```python
from build123d import *

# Parameters (mm, degrees)
F0_R     = 12.7
F1_DEPTH = 19.05
F2_DEPTH = 6.35
F0_R_2   = 4.7625
F3_DEPTH = 9.525


with BuildPart() as f1:
    # F0 (on Front) → F1 (new body)
    with BuildSketch(Plane.XZ):
        with BuildLine():
            Line((21.9405616204, -3.5443449016), (22.1211236947, -2.1462785193))
            ThreePointArc((22.1211236947, -2.1462785193), (22.199015734, -1.0743953845), (22.225, 0))
            Line((22.225, 0), (21.5661626468, 5.3713363041))
            ThreePointArc((21.5661626468, 5.3713363041), (-1.3190436674, 22.1858231491), (-22.0506835685, 2.7781251166))
            ThreePointArc((-22.0506835685, 2.7781251166), (-22.225, 1.708e-07), (-22.0506836112, -2.7781247776))
            ThreePointArc((-22.0506836112, -2.7781247776), (-0.3870465512, -22.2216295525), (21.9405616204, -3.5443449016))
        make_face()
        Circle(F0_R, mode=Mode.SUBTRACT)
    extrude(amount=F1_DEPTH)

    # F0 (on Front) → F2 (join)
    with BuildSketch(Plane.XZ):
        with BuildLine():
            ThreePointArc((-22.0506835685, 2.7781251166), (-1.3190436674, 22.1858231491), (21.5661626468, 5.3713363041))
            Line((21.5661626468, 5.3713363041), (15.7569112616, 52.732711177))
            ThreePointArc((15.7569112616, 52.732711177), (15.8454503135, 51.7681577149), (15.875, 50.8))
            ThreePointArc((15.875, 50.8), (-0.9941387366, 34.9561585096), (-15.7504882737, 52.784375))
            Line((-15.7504882737, 52.784375), (-22.0506835685, 2.7781251166))
        make_face()
        with BuildLine():
            Line((15.8726570063, -50.5272646713), (21.9405616204, -3.5443449016))
            ThreePointArc((21.9405616204, -3.5443449016), (-0.3870465512, -22.2216295525), (-22.0506836112, -2.7781247776))
            Line((-22.0506836112, -2.7781247776), (-15.7504882737, -52.784375))
            ThreePointArc((-15.7504882737, -52.784375), (-1.1302070867, -34.9652831746), (15.8726570063, -50.5272646713))
        make_face()
    extrude(amount=F2_DEPTH)

    # F0 (on Front) → F3 (join)
    with BuildSketch(Plane.XZ):
        with BuildLine():
            ThreePointArc((15.875, 50.8), (15.8454503135, 51.7681577149), (15.7569112616, 52.732711177))
            ThreePointArc((15.7569112616, 52.732711177), (0.0260307769, 66.6749786582), (-15.7504882737, 52.784375))
            ThreePointArc((-15.7504882737, 52.784375), (-0.9941387366, 34.9561585096), (15.875, 50.8))
        make_face()
        with Locations((0, 50.8)):
            Circle(F0_R_2, mode=Mode.SUBTRACT)
        with BuildLine():
            ThreePointArc((15.875, -50.8), (15.8744142408, -50.6636273038), (15.8726570063, -50.5272646713))
            ThreePointArc((15.8726570063, -50.5272646713), (-1.1302070867, -34.9652831746), (-15.7504882737, -52.784375))
            ThreePointArc((-15.7504882737, -52.784375), (0.9941387366, -66.6438414904), (15.875, -50.8))
        make_face()
        with Locations((0, -50.8)):
            Circle(F0_R_2, mode=Mode.SUBTRACT)
    extrude(amount=F3_DEPTH)


solid = f1.part
```
For this review, take the finished solid that the model builds, in its own axes (mm). A direction names the side the tool comes from. Give positions to 0.01 mm unless a question says otherwise; leave off trailing zeros. Order: outer loops, then holes, each group sorted by start corner. A loop starts at its lowest first (then second) coordinate and runs counter-clockwise, first axis right, second up.
1) Take a section at D-D (y = -17). Give the boundary of the cut face in (x, z) (3 decimals), then the cut area to 3 significant figures.
2) The part is to be moulded in two halves that separate along Z. For faces 1 (the face through (-1.03, -4.7, -55.45)), 2 (the face through (-2.75, -9.39, -12.4)), 3 (the face through (19.755, -5.158, 20.138)), 4 (the face through (10, -19.05, -10)), say which applies: released by +Z, released by -Z, zero draft, split by the parting line, or undercut.
3) Take a section at C-C (z = 18). Give the boundary of the cut face in (x, y), then the cut area to 3 significant figures.
4) Insertion check: pin 1 (3 mm diameter, centred on y = -3.5, z = -34.5, fed in from +X); pin 2 (6 mm diameter, centred on y = -8, z = -31, fed in from -X); pin 3 (13 mm diameter, centred on x = -0.5, z = -31, fed in from -Y) (3 decimals). Each pin has a flat end and moves straight along its axis. Give the tip position at first contact, or say it passes through.
5) For faces 5 (the face through (3.3, -9.525, -47)), 6 (the face through (3, -9.525, 55)), 7 (the face through (0, -6.35, 30)), list the 3-axis set-ups (+Z, -Z, +X, -X, +Y, -Y) from which the entire face can be reached by the end or side of a thin tool; tool diameter is ignored.
6) Wall thickness on line 1 (Z direction, x = 0, y = -5.5) (1 decimal); line 2 (Y direction, x = -11.5, z = -24.5); line 3 (X direction, y = -2.5, z = 10): over which ranges is each line inside the solid? List them lowest first.
7) Take a section at A-A (x = 0). State how many separate pieces and enclosed holes the cut face has, then the cut area to 3 significant figures.
Derived:
1. outline: (21.566, 5.371) arc R22.225 ccw (long way) to (21.941, -3.544) - (22.121, -2.146) arc R22.225 ccw to (22.225, 0) - close; hole circle Ø25.4 at (0, 0)
1. area: 1,040 mm2
2. face 1: undercut
2. face 2: undercut
2. face 3: released by +Z
2. face 4: zero draft
3. outline: (-20.13, -6.35) - (-13.04, -6.35) - (-13.04, -19.05) - (13.04, -19.05) - (13.04, -6.35) - (20.02, -6.35) - (20.02, 0) - (-20.13, 0) - close
3. area: 586 mm2
4. pin 1: stops at x = 18.14
4. pin 2: stops at x = -18.81
4. pin 3: stops at y = -9.525
5. face 5: -Z, +X, -X, -Y
5. face 6: +Z, +X, -X, -Y
5. face 7: -Y
6. line 1: z = -66.7 to -55.6, -46 to -12.7, 12.7 to 46, 55.6 to 66.7
6. line 2: y = -6.35 to 0
6. line 3: x = -21.14 to -7.83, 7.83 to 21
7. separate pieces: 4
7. enclosed holes: 0
7. area: 948 mm2
